Part print with two shaded views. Sizes in mm from the minimum x, y, z corner. A direction names the side the tool comes from. Give positions to 0.01 mm unless a question says otherwise; leave off trailing zeros. Order: outer loops, then holes, each group sorted by start corner. A loop starts at its lowest first (then second) coordinate and runs counter-clockwise, first axis right, second up. Notation, with made-up numbers: (-33, -30.75) -> (26, -30.75) arc R22 cw to (26, -13.75) -> close; hole circle Ø6 at (9.25, 33.5). An arc over 180 degrees is marked (long way). Write item = value, one per line. Start each with the question number.
Item 1: Band-saw the part on C-C on x = 9. Write the cut outline in (y, z), plus the area to 3 significant figures.
Item 2: Pull direction X, two halves, no side cores. Call the marked faces 3, 4 and 5: +X half, -X half, draft (parallel to the pull), parting line (faces both ways), or undercut.
Item 3: Drill centre lines: line 1 along Z through (x, y) = (26.5, 6.5); line 2 along Z through (x, y) = (26, 1); line 3 along X through (y, z) = (17, 26). Where is each one in solid material? Low to high.
Item 4: Band-saw the part on B-B on y = 23. Write the cut outline in (x, z).
Item 5: Flat gauge pins, fed straight in: P1, Ø1.5, axis at x = 21.5, y = 28.5, coming from the -Z side; P2, Ø15, axis at x = 24, z = 24.5, coming from the +Y side; P3, Ø12, axis at x = 19, y = 7, coming from the +Z side; P4, Ø8, axis at x = 26, z = 26, coming from the -Y side. Where does each tip first touch, or does it go through?
Item 6: Band-saw the part on D-D on x = 26. Count the separate pieces of the cut face and the enclosed holes in it, plus the area to 3 significant figures.
Item 7: Tool access for the marked faces 1 and 2: list every direction of +Z, -Z, +X, -X, +Y, -Y with a clear straight run to the whole face (end or side of a thin tool).
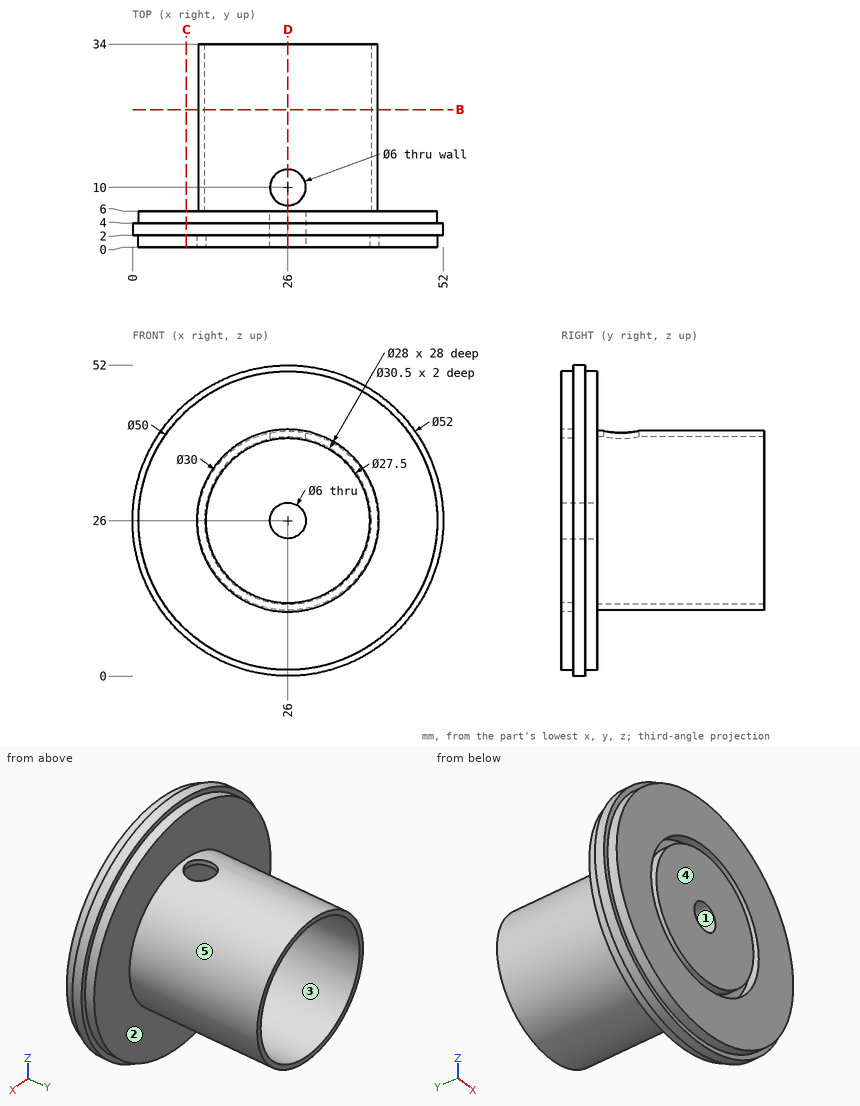
Values found:
q1.outline = (0, 7.67) -> (2, 7.67) -> (2, 6.33) -> (4, 6.33) -> (4, 7.67) -> (6, 7.67) -> (6, 44.33) -> (4, 44.33) -> (4, 45.67) -> (2, 45.67) -> (2, 44.33) -> (0, 44.33) -> close
q1.area = 225 mm^2
q2.face_3 = undercut
q2.face_4 = draft
q2.face_5 = parting line
q3.line_1 = 11.01 to 12.01, 39.99 to 40.99
q3.line_2 = 1 to 10.75, 12.25 to 23, 29 to 39.75, 41.25 to 51
q3.line_3 = 11 to 12, 40 to 41
q4.outline = circle Ø30 at (26, 26); hole circle Ø28 at (26, 26)
q5.P1 = 11.48
q5.P2 = 6
q5.P3 = 51.94
q5.P4 = 0
q6.separate_pieces = 3
q6.enclosed_holes = 0
q6.area = 312 mm^2
q7.face_1 = +Y, -Y
q7.face_2 = +Y
